Input: part model. Units: mm. Frame: model coordinates. Face numbers are marked on the shaded views. A direction names the side the tool comes from. Give positions to 0.01 mm unless a question says otherwise; leave off trailing zeros. Write each loop counter-clockwise with the first axis right and the second up, starting at its lowest first coordinate (ties: lowest second). Pieces come first, ordered by that corner, then holes. Notation, with made-up numbers: (78, -6) - (112, -6) arc R16 cw to (112, -2) - close; hole circle Ø8 at (-7.75, -39.5). An arc over 180 degrees is marked (long way). Use a Markdown table: item, result. Add a question column.
1. Pin query (flat end, axial travel): pin 1 (1.5 mm diameter, centred on x = -91.5, z = 49.5, fed in from +Y); pin 2 (1 mm diameter, centred on x = 159.5, z = 116, fed in from +Y); pin 3 (5 mm diameter, centred on x = 16, z = 46.5, fed in from +Y). Return the tip coordinate at first contact, or that it passes through.
2. Section query D-D, the plane z = 104. Return loops of the section in (x, y), plus the area to 3 significant figures.
3. Material intervals for probe 1 along Y at (x, z) = (235, 96); probe 2 along X at (y, z) = (101, 119.5); probe 3 along Z at (x, y) = (165, 49), sorted ascending.
4. Section query C-C, the plane z = 27.5. Return loops of the section in (x, y), plus the area to 3 significant figures.
5. Section query B-B, the plane x = 29.5. Return loops of the section in (y, z).
6. Set-up query: the marked faces 1, 2, 3, 4 and 5. Return all of +Z, -Z, +X, -X, +Y, -Y with unobstructed straight access to the full face (end or side cutting, diameter ignored); none if empty.
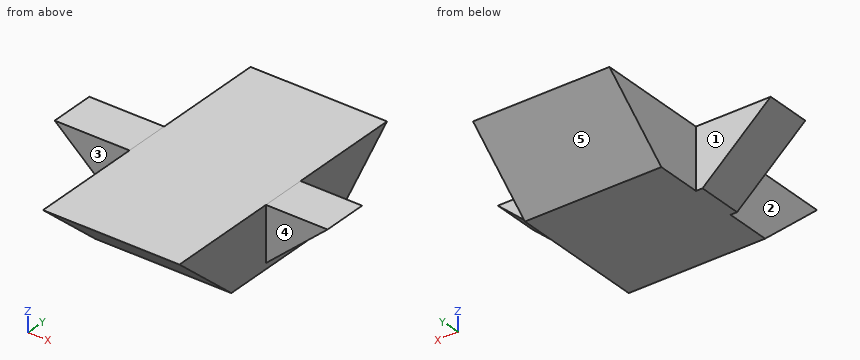
```python
from build123d import *

# Parameters (mm, degrees)
F1_DEPTH = 50.8
F3_DEPTH = 152.4


with BuildPart() as f1:
    # F0 (on Front) → F1 (new body, symmetric)
    with BuildSketch(Plane.XZ):
        Polygon((0, 134.4041666021), (-319.4691668987, 134.4041666021), (-167.0691668987, 0), (0, 0), align=None)
        Polygon((290.1308331013, 134.4041666021), (0, 134.4041666021), (0, 0), (137.7308331013, 0), align=None)
    extrude(amount=F1_DEPTH, both=True)

    # F2 (on Right) → F3 (join, symmetric)
    with BuildSketch(Plane.YZ):
        Polygon((-152.4, 0), (0, 0), (0, 134.4041762), (-304.8, 134.4041762), align=None)
        Polygon((0, 134.4041762), (0, 0), (152.4, 0), (304.8, 134.4041762), align=None)
    extrude(amount=F3_DEPTH, both=True)


solid = f1.part
```
Result sheet:
| question | item | result |
|---|---|---|
| 1 | pin 1 | stops at y = 209.38 |
| 1 | pin 2 | stops at y = 50.8 |
| 1 | pin 3 | stops at y = 207.96 |
| 2 | outline | (-284.99, -50.8) - (-152.4, -50.8) - (-152.4, -270.32) - (152.4, -270.32) - (152.4, -50.8) - (255.66, -50.8) - (255.66, 50.8) - (152.4, 50.8) - (152.4, 270.32) - (-152.4, 270.32) - (-152.4, 50.8) - (-284.99, 50.8) - close |
| 2 | area | 189,000 mm² |
| 3 | probe 1 | y = -50.8 to 50.8 |
| 3 | probe 2 | x = -152.4 to 152.4 |
| 3 | probe 3 | z = 24.05 to 134.4 |
| 4 | outline | (-198.25, -50.8) - (-152.4, -50.8) - (-152.4, -183.58) - (152.4, -183.58) - (152.4, -50.8) - (168.91, -50.8) - (168.91, 50.8) - (152.4, 50.8) - (152.4, 183.58) - (-152.4, 183.58) - (-152.4, 50.8) - (-198.25, 50.8) - close |
| 4 | area | 118,000 mm² |
| 5 | outline | (-304.8, 134.4) - (-152.4, 0) - (152.4, 0) - (304.8, 134.4) - close |
| 6 | face 1 | +Z, -Z, -X, +Y |
| 6 | face 2 | +Z, -Z, -X, -Y |
| 6 | face 3 | +Z, -Z, -X, -Y |
| 6 | face 4 | +Z, -Z, +X, -Y |
| 6 | face 5 | -Z, +X, -X, +Y |
